Autodesk Inventor part; units mm, degrees
ref_plane "YZ Plane" through (0, 0, 0) normal (1, 0, 0) x (0, 1, 0)
ref_plane "XZ Plane" through (0, 0, 0) normal (0, 1, 0) x (-1, 0, 0)
ref_plane "XY Plane" through (0, 0, 0) normal (0, 0, 1) x (1, 0, 0)
sketch "Sketch1" plane through (0, 0, 0) normal (0, 1, 0) x (-1, 0, 0)
  line L0 (0, 0) -> (0, -133.35)
  line L1 (0, -133.35) -> (41.275, -133.35)
  line L2 (41.275, -133.35) -> (41.275, 0)
  line L3 (41.275, 0) -> (0, 0)
  dimension "d0" = 133.35
  dimension "d1" = 41.275
extrude "Extrusion1" add sketch "Sketch1" along normal blind 3.175
sketch "Sketch2" plane through (0, 3.175, 0) normal (0, 1, 0) x (1, 0, 0)
  line L0 (-41.275, 133.35) -> (-41.275, 0)
  line L1 (-41.275, 0) -> (-38.1, 0)
  line L2 (-41.275, 0) -> (0, 0)
  line L3 (-38.1, 0) -> (-38.1, 133.35)
  line L4 (0, 133.35) -> (-41.275, 133.35)
  line L5 (-41.275, 133.35) -> (-41.275, 0)
  dimension "d4" = 3.175
extrude "Extrusion2" add sketch "Sketch2" along normal blind 38.1
sketch "Sketch3" plane through (0, 41.275, 0) normal (0, 1, 0) x (1, 0, 0)
  line L0 (-41.275, 133.35) -> (-41.275, 0)
  line L1 (-41.275, 66.675) -> (-41.275, 84.1375)
  line L2 (-41.275, 66.675) -> (-41.275, 49.1998)
  line L3 (-41.275, 49.1998) -> (-38.1, 49.1998)
  line L4 (-38.1, 0) -> (-38.1, 133.35)
  line L5 (-38.1, 84.1375) -> (-41.275, 84.1375)
  line L6 (-38.1, 49.1998) -> (-38.1, 84.1375)
  point P0 (0, 0)
  dimension "d7" = 17.4625
  dimension "d8" = 17.4752
extrude "Extrusion3" cut sketch "Sketch3" against normal blind 25.4
sketch "Sketch4" plane through (0, 3.175, 0) normal (0, 1, 0) x (1, 0, 0)
  line L0 (0, 133.35) -> (-38.1, 133.35)
  point P0 (0, 0)
sketch "Sketch5" plane through (0, 3.175, 0) normal (0, 1, 0) x (1, 0, 0)
  line L0 (0, 0) -> (0, 133.35)
  line L1 (0, 66.675) -> (-38.3992, 66.675)
  line L2 (-19.1996, 66.675) -> (-19.1996, 118.0846)
  line L3 (-19.1996, 66.675) -> (-19.1996, 15.2654)
  circle A0 centre (-19.1996, 15.2654) radius 1.905
  circle A1 centre (-19.1996, 118.0846) radius 1.905
  dimension "d12" = 51.4096
  dimension "d13" = 51.4096
  dimension "d14" = 3.81
  dimension "d15" = 3.81
extrude "Extrusion4" cut sketch "Sketch5" against normal blind 20.6375
properties part number "cut top wheel mout thingy"
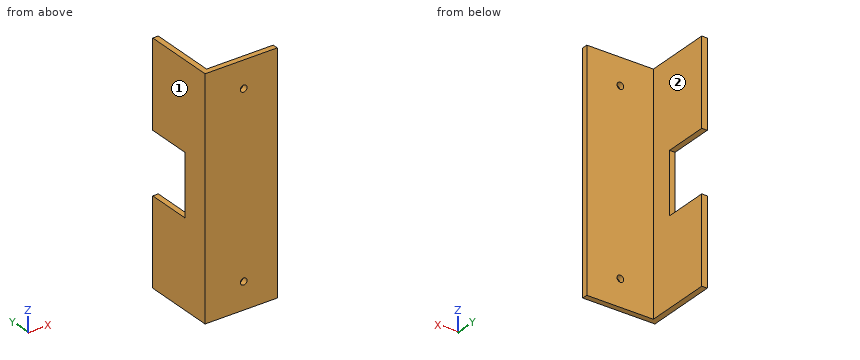
Could you check a few things on this model? Use its own coordinates, in mm. Face numbers are marked on the shaded views. A direction names the side the tool comes from. Round coordinates to 2 decimals unless told otherwise and drop trailing zeros. Loops run counter-clockwise (first coordinate to the right, second up) from the corner with the lowest first, then second, coordinate; pieces in that order, holes last. Notation, with made-up numbers: (66, 35.25) - (106, 35.25) arc R31 ccw to (106, 65.25) - close; hole circle Ø6 at (2.25, 73). An arc over 180 degrees is marked (long way). Write item = value, one per line.
1) Imagine slicing it at C-C (x = -31). Please give me the cut outline in (y, z) (3 decimals), and give its area (3 significant figures).
Computed:
outline = (0, -133.35) - (3.175, -133.35) - (3.175, 0) - (0, 0) - close
area = 423 mm2
2) I need wall thicknesses on line 1 along Y through (x, z) = (-5, -79.5) (3 decimals); line 2 along X through (y, z) = (28.5, -92.5) (3 decimals). Which ranges of each line are inside material? Lowest first, please. Write a range as from..to.
Computed:
line_1 = 0..3.175
line_2 = -41.275..-38.1
3) On a 3-axis mill with a long thin cutter (end or side, diameter ignored), from which of +Z, -Z, +X, -X, +Y, -Y can I reach the whole of each face in a straight line? I mean the marked faces 1 and 2. Say none if no direction works.
Computed:
face_1 = +Z, -Z, -X, +Y, -Y
face_2 = +Z, -Z, +X, +Y
4) Imagine slicing it at B-B (z = -79). Please give me the cut outline in (x, y) (3 decimals), and give its area (3 significant figures).
Computed:
outline = (-41.275, 0) - (0, 0) - (0, 3.175) - (-38.1, 3.175) - (-38.1, 15.875) - (-41.275, 15.875) - close
area = 171 mm2
5) I'm going to push flat-ended pins straight in: P1, Ø11.5, axis at y = 25.5, z = -40, coming from the +X side; P2, Ø1.6, axis at x = -40.5, z = -70, coming from the +Y side (3 decimals); P3, Ø3, axis at x = -28.5, z = -71, coming from the +Y side (3 decimals). Where does each tip first touch, or does it pass through?
Computed:
P1 = -38.1
P2 = 15.875
P3 = 3.175
6) Imagine slicing it at D-D (z = -28.5). Please give me the cut outline in (x, y) (3 decimals).
Computed:
outline = (-41.275, 0) - (0, 0) - (0, 3.175) - (-38.1, 3.175) - (-38.1, 41.275) - (-41.275, 41.275) - close
